Read the model definition and answer for the solid it produces. Units are mm, in the model's axes. Face numbers are marked on the shaded views. A direction names the side the tool comes from. Coordinates: 2 decimals unless noted, no trailing zeros. Answer in a Markdown table with one row per item.
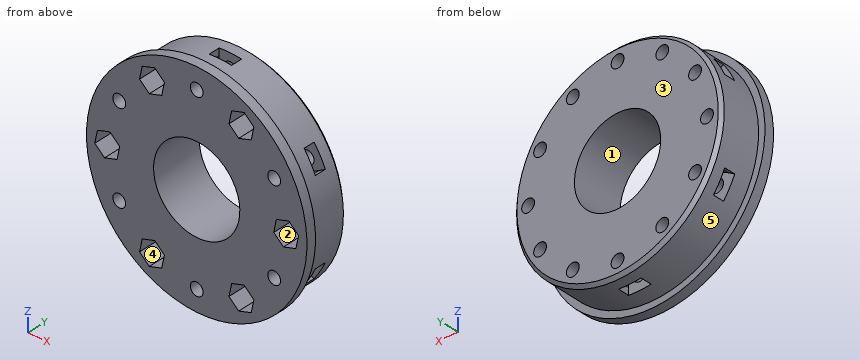
from build123d import *

# Parameters (mm, degrees)
SKETCH_1_R          = 34.5
EXTRUDE_1_DEPTH     = 16
CUT_EXTRUDE_START   = -13
SKETCH_2_R          = 34.5
SKETCH_2_R_2        = 32.5
CUT_EXTRUDE_1_DEPTH = 13
SKETCH_3_R          = 2
CUT_EXTRUDE_3_DEPTH = 52.34685969
SKETCH_7_R          = 13.5
CUT_EXTRUDE_6_DEPTH = 52.34685969
CUT_EXTRUDE_7_DEPTH = 8
CHAMFER_4_SIZE      = 1
CUT_EXTRUDE_8_DEPTH = 1.75
CUT_EXTRUDE_9_REACH = 53.347
SKETCH_11_R         = 2


with BuildPart() as part:
    # 草图1 → 凸台-拉伸1 (new body)
    with BuildSketch(Plane(origin=(0, 0, 0), x_dir=(1, 0, 0), z_dir=(0, 1, 0))):
        with Locations(Location((0, 0, 0), (0, 0, 270))):
            Circle(SKETCH_1_R)
    extrude(amount=EXTRUDE_1_DEPTH)

    # 草图2 → 切除-拉伸1 (cut)
    with BuildSketch(Plane(origin=(0, 16, 0), x_dir=(1, 0, 0), z_dir=(0, 1, 0)).offset(CUT_EXTRUDE_START)):
        with Locations(Location((0, 0, 0), (0, 0, 270))):
            Circle(SKETCH_2_R)
        with Locations(Location((0, 0, 0), (0, 0, 270))):
            Circle(SKETCH_2_R_2, mode=Mode.SUBTRACT)
    extrude(amount=CUT_EXTRUDE_1_DEPTH, mode=Mode.SUBTRACT)

    # 草图3 → 切除-拉伸3 (cut, through all)
    with BuildSketch(Plane(origin=(0, 16, 0), x_dir=(1, 0, 0), z_dir=(0, 1, 0))):
        with Locations(Location((-28, 0, 0), (0, 0, 270))):
            Circle(SKETCH_3_R)
        with Locations(Location((-14, 24.248711306, 0), (0, 0, 270))):
            Circle(SKETCH_3_R)
        with Locations(Location((14, 24.248711306, 0), (0, 0, 270))):
            Circle(SKETCH_3_R)
        with Locations(Location((28, 0, 0), (0, 0, 270))):
            Circle(SKETCH_3_R)
        with Locations(Location((14, -24.248711306, 0), (0, 0, 270))):
            Circle(SKETCH_3_R)
        with Locations(Location((-14, -24.248711306, 0), (0, 0, 270))):
            Circle(SKETCH_3_R)
    extrude(amount=-CUT_EXTRUDE_3_DEPTH, mode=Mode.SUBTRACT)

    # 草图7 → 切除-拉伸6 (cut, through all)
    with BuildSketch(Plane(origin=(0, 16, 0), x_dir=(1, 0, 0), z_dir=(0, 1, 0))):
        with Locations(Location((0, 0, 0), (0, 0, 270))):
            Circle(SKETCH_7_R)
    extrude(amount=-CUT_EXTRUDE_6_DEPTH, mode=Mode.SUBTRACT)

    # 草图8 → 切除-拉伸7 (cut)
    with BuildSketch(Plane.XZ):
        Polygon((14.841047387, -20.236732664), (10.94604827, -21.514353582), (10.105000883, -25.526332224), (13.158952613, -28.260689948), (17.05395173, -26.98306903), (17.894999117, -22.971090388), align=None)
        Polygon((31.894999117, 1.277620918), (28.841047387, 4.011978642), (24.94604827, 2.734357724), (24.105000883, -1.277620918), (27.158952613, -4.011978642), (31.05395173, -2.734357724), align=None)
        Polygon((-10.105000883, -22.971090388), (-13.158952613, -20.236732664), (-17.05395173, -21.514353582), (-17.894999117, -25.526332224), (-14.841047387, -28.260689948), (-10.94604827, -26.98306903), align=None)
        Polygon((-24.94604827, -2.734357724), (-24.105000883, 1.277620918), (-27.158952613, 4.011978642), (-31.05395173, 2.734357724), (-31.894999117, -1.277620918), (-28.841047387, -4.011978642), align=None)
        Polygon((-14.841047387, 20.236732664), (-10.94604827, 21.514353582), (-10.105000883, 25.526332224), (-13.158952613, 28.260689948), (-17.05395173, 26.98306903), (-17.894999117, 22.971090388), align=None)
        Polygon((10.105000883, 22.971090388), (13.158952613, 20.236732664), (17.05395173, 21.514353582), (17.894999117, 25.526332224), (14.841047387, 28.260689948), (10.94604827, 26.98306903), align=None)
    extrude(amount=-CUT_EXTRUDE_7_DEPTH, mode=Mode.SUBTRACT)

    # 倒角4
    chamfer_4_edges = [part.edges().sort_by_distance(p)[0] for p in [
        (0, 16, -32.5),
    ]]
    chamfer(chamfer_4_edges, length=CHAMFER_4_SIZE)

    # 草图10 → 切除-拉伸8 (cut, symmetric)
    with BuildSketch(Plane(origin=(0, 10, 0), x_dir=(1, 0, 0), z_dir=(0, 1, 0))):
        Polygon((-3.482371577, -30.162503534), (-3.613968785, -26.065429516), (-0.131597208, -23.902925982), (3.482371577, -25.837496466), (3.613968785, -29.934570484), (3.482371577, -34.323797695), (-3.482371577, -34.323797695), align=None)
        Polygon((-27.86268009, -12.065429516), (-24.380308514, -9.902925982), (-20.766339729, -11.837496466), (-20.634742521, -15.934570484), (-24.117114098, -18.097074018), (-27.98409497, -20.177721098), (-31.466466547, -14.146076596), align=None)
        Polygon((-24.380308514, 18.097074018), (-20.766339729, 16.162503534), (-20.634742521, 12.065429516), (-24.117114098, 9.902925982), (-27.731082883, 11.837496466), (-31.466466547, 14.146076596), (-27.98409497, 20.177721098), align=None)
        Polygon((3.482371577, 30.162503534), (3.613968785, 26.065429516), (0.131597208, 23.902925982), (-3.482371577, 25.837496466), (-3.613968785, 29.934570484), (-3.482371577, 34.323797695), (3.482371577, 34.323797695), align=None)
        Polygon((27.86268009, 12.065429516), (24.380308514, 9.902925982), (20.766339729, 11.837496466), (20.634742521, 15.934570484), (24.117114098, 18.097074018), (27.98409497, 20.177721098), (31.466466547, 14.146076596), align=None)
        Polygon((24.380308514, -18.097074018), (20.766339729, -16.162503534), (20.634742521, -12.065429516), (24.117114098, -9.902925982), (27.731082883, -11.837496466), (31.466466547, -14.146076596), (27.98409497, -20.177721098), align=None)
    extrude(amount=CUT_EXTRUDE_8_DEPTH, both=True, mode=Mode.SUBTRACT)

    # 切除-拉伸9: up to this face of the body (flat: up to its plane)
    cut_extrude_9_end = Plane(part.part.faces().sort_by_distance((0, 16, -30.609045456))[0])
    # 草图11 → 切除-拉伸9 (cut, up to the picked face)
    with BuildSketch(Plane.XZ, mode=Mode.PRIVATE) as cut_extrude_9_sk1:
        with Locations(Location((0, 28, 0), (0, 0, 270))):
            Circle(SKETCH_11_R)
    cut_extrude_9_tool1 = split(extrude(cut_extrude_9_sk1.sketch, amount=-CUT_EXTRUDE_9_REACH, mode=Mode.PRIVATE), bisect_by=cut_extrude_9_end, keep=Keep.BOTH, mode=Mode.PRIVATE)
    # 草图11 → 切除-拉伸9 (cut, up to the picked face)
    with BuildSketch(Plane.XZ, mode=Mode.PRIVATE) as cut_extrude_9_sk2:
        with Locations(Location((24.248711306, 14, 0), (0, 0, 270))):
            Circle(SKETCH_11_R)
    cut_extrude_9_tool2 = split(extrude(cut_extrude_9_sk2.sketch, amount=-CUT_EXTRUDE_9_REACH, mode=Mode.PRIVATE), bisect_by=cut_extrude_9_end, keep=Keep.BOTH, mode=Mode.PRIVATE)
    # 草图11 → 切除-拉伸9 (cut, up to the picked face)
    with BuildSketch(Plane.XZ, mode=Mode.PRIVATE) as cut_extrude_9_sk3:
        with Locations(Location((24.248711306, -14, 0), (0, 0, 270))):
            Circle(SKETCH_11_R)
    cut_extrude_9_tool3 = split(extrude(cut_extrude_9_sk3.sketch, amount=-CUT_EXTRUDE_9_REACH, mode=Mode.PRIVATE), bisect_by=cut_extrude_9_end, keep=Keep.BOTH, mode=Mode.PRIVATE)
    # 草图11 → 切除-拉伸9 (cut, up to the picked face)
    with BuildSketch(Plane.XZ, mode=Mode.PRIVATE) as cut_extrude_9_sk4:
        with Locations(Location((0, -28, 0), (0, 0, 270))):
            Circle(SKETCH_11_R)
    cut_extrude_9_tool4 = split(extrude(cut_extrude_9_sk4.sketch, amount=-CUT_EXTRUDE_9_REACH, mode=Mode.PRIVATE), bisect_by=cut_extrude_9_end, keep=Keep.BOTH, mode=Mode.PRIVATE)
    # 草图11 → 切除-拉伸9 (cut, up to the picked face)
    with BuildSketch(Plane.XZ, mode=Mode.PRIVATE) as cut_extrude_9_sk5:
        with Locations(Location((-24.248711306, -14, 0), (0, 0, 270))):
            Circle(SKETCH_11_R)
    cut_extrude_9_tool5 = split(extrude(cut_extrude_9_sk5.sketch, amount=-CUT_EXTRUDE_9_REACH, mode=Mode.PRIVATE), bisect_by=cut_extrude_9_end, keep=Keep.BOTH, mode=Mode.PRIVATE)
    # 草图11 → 切除-拉伸9 (cut, up to the picked face)
    with BuildSketch(Plane.XZ, mode=Mode.PRIVATE) as cut_extrude_9_sk6:
        with Locations(Location((-24.248711306, 14, 0), (0, 0, 270))):
            Circle(SKETCH_11_R)
    cut_extrude_9_tool6 = split(extrude(cut_extrude_9_sk6.sketch, amount=-CUT_EXTRUDE_9_REACH, mode=Mode.PRIVATE), bisect_by=cut_extrude_9_end, keep=Keep.BOTH, mode=Mode.PRIVATE)
    add(cut_extrude_9_tool1.solids().sort_by(Axis((0, 0, 28), (0, 1, 0)))[0], mode=Mode.SUBTRACT)
    add(cut_extrude_9_tool2.solids().sort_by(Axis((24.248711, 0, 14), (0, 1, 0)))[0], mode=Mode.SUBTRACT)
    add(cut_extrude_9_tool3.solids().sort_by(Axis((24.248711, 0, -14), (0, 1, 0)))[0], mode=Mode.SUBTRACT)
    add(cut_extrude_9_tool4.solids().sort_by(Axis((0, 0, -28), (0, 1, 0)))[0], mode=Mode.SUBTRACT)
    add(cut_extrude_9_tool5.solids().sort_by(Axis((-24.248711, 0, -14), (0, 1, 0)))[0], mode=Mode.SUBTRACT)
    add(cut_extrude_9_tool6.solids().sort_by(Axis((-24.248711, 0, 14), (0, 1, 0)))[0], mode=Mode.SUBTRACT)


solid = part.part
Q1. Consider line 1 (Y direction, x = -26, z = 15.5); line 2 (Z direction, x = 2, y = 11.25); line 3 (Z direction, x = -22, y = 8.5). Determine where each line is inside the solid, lowest interval first.
Outcome:
| item | result |
|---|---|
| line 1 | 0 to 8.25, 11.75 to 16 |
| line 2 | -25.06 to -13.35, 13.35 to 25.04 |
| line 3 | -23.92 to -16.82, -11.22 to 11.18, 16.78 to 23.92 |
Q2. For a pull along Z with two mould halves and no side action, classify the marked faces 3, 4 and 5 as pulls with the +Z half, pulls with the -Z half, needs draft (parallel to the pull), parting line crosses it, or undercut.
Outcome:
| item | result |
|---|---|
| face 3 | needs draft |
| face 4 | undercut |
| face 5 | parting line crosses it |
Q3. For the marked faces 1 and 2, determine the directions among +Z, -Z, +X, -X, +Y, -Y from which every point of the face is accessible in a straight line to the end or side of a thin tool.
Outcome:
| item | result |
|---|---|
| face 1 | +Y, -Y |
| face 2 | -Y |
Q4. The part is cut by section A-A (y = 13). Give the number of separate pieces and of enclosed holes in the cut face, then the cut area to 3 significant figures.
Outcome:
| item | result |
|---|---|
| separate pieces | 1 |
| enclosed holes | 13 |
| area | 2,590 mm² |
Q5. Given pin 1 (21.5 mm diameter, centred on x = 0, z = 0, fed in from +Y); pin 2 (8.5 mm diameter, centred on x = -13, z = 23.5, fed in from -Y); pin 3 (1 mm diameter, centred on x = 12.5, y = 9.5, fed in from -Z); pin 4 (5 mm diameter, centred on y = 10, z = -6, fed in from -X), each flat-ended and moving along its own axis, determine where each tip first touches the part or whether it passes through.
Outcome:
| item | result |
|---|---|
| pin 1 | through |
| pin 2 | y = 0 |
| pin 3 | z = -30.2 |
| pin 4 | x = -32.31 |
